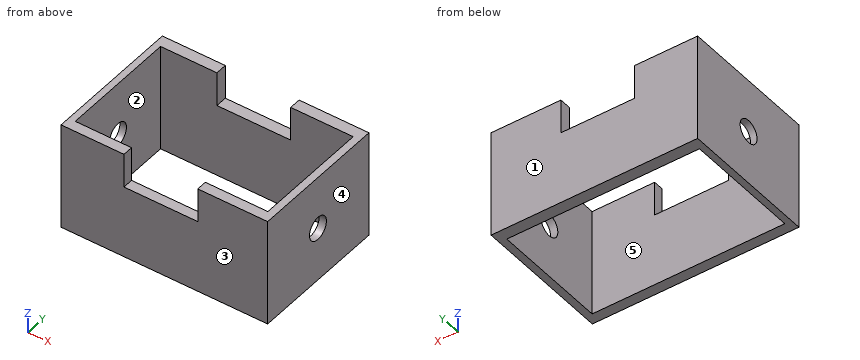
```python
from build123d import *

# Parameters (mm, degrees)
F0_W     = 219.245888
F0_H     = 147.08846
F1_DEPTH = 114.3
F2_W     = 78.317389
F2_H     = 36.511922
F3_DEPTH = 147.089461
F4_W     = 204.472921
F4_H     = 123.958089
F5_DEPTH = 114.301
F6_R     = 12.264791
F7_DEPTH = 219.246888


with BuildPart() as f1:
    # F0 (on Top) → F1 (new body)
    with BuildSketch(Plane.XY):
        with Locations((10.201607, 0.449974)):
            Rectangle(F0_W, F0_H)
    extrude(amount=F1_DEPTH)

    # F2 (on face) → F3 (cut, through all)
    with BuildSketch(Plane.XZ.offset(73.094256)):
        with Locations((6.517709, 96.044039)):
            Rectangle(F2_W, F2_H)
    extrude(amount=-F3_DEPTH, mode=Mode.SUBTRACT)

    # F4 (on face) → F5 (cut, through all)
    with BuildSketch(Plane(origin=(0, 0, 0), x_dir=(1, 0, 0), z_dir=(0, 0, -1))):
        with Locations((9.806979, 0.144809)):
            Rectangle(F4_W, F4_H)
    extrude(amount=-F5_DEPTH, mode=Mode.SUBTRACT)

    # F6 (on face) → F7 (cut, through all)
    with BuildSketch(Plane.YZ.offset(119.824551)):
        with Locations((0, 57.527971)):
            Circle(F6_R)
    extrude(amount=-F7_DEPTH, mode=Mode.SUBTRACT)


solid = f1.part
```
Model file for the job. Use its own axes, mm. Face numbers are marked on the shaded views. A direction names the side the tool comes from. Coordinates: 2 decimals unless noted, no trailing zeros. Order: outer loops, then holes, each group sorted by start corner. A loop starts at its lowest first (then second) coordinate and runs counter-clockwise, first axis right, second up. Notation, with made-up numbers: (75.5, 35.25) - (123.5, 35.25) arc R9 cw to (123.5, 39.25) - close; hole circle Ø9 at (46.25, 65). An arc over 180 degrees is marked (long way). Return JSON: item names as keys, results as strings. Group by question number.
1) Saw through at C-C, the plane z = 75. Write the cut outline in (x, y).
2) Tool access for the marked faces 1 and 2: list every direction of +Z, -Z, +X, -X, +Y, -Y with a clear straight run to the whole face (end or side of a thin tool).
3) Mould opens along X. For the marked faces 3, 4 and 5 say: released by +X, released by -X, zero draft, split by the parting line, or undercut.
4) Saw through at D-D, the plane y = -19. Write the cut outline in (x, z).
5) Probe line 1 (Y direction, x = -80, z = 53); line 2 (X direction, y = -26, z = 67); line 3 (Z direction, x = -96, y = 0). List the from-to ranges inside material, lowest first. Write a range as from..to.
6) Saw through at A-A, the plane y = 0. Write the cut outline in (x, z).
7) Saw through at B-B, the plane x = 74.5. Write the cut outline in (y, z).
8) Flat gauge pin, fed straight in: P1, Ø3.5, axis at x = -8, y = 66, coming from the +Z side. Where does the tip first touch, or does it go through?
Values found:
{
 "1": {"outline": "(-99.42, -73.09) - (119.82, -73.09) - (119.82, 73.99) - (-99.42, 73.99) - close; hole (-92.43, -62.12) - (112.04, -62.12) - (112.04, 61.83) - (-92.43, 61.83) - close"},
 "2": {"face 1": "+Z, -Z, +X, -X, +Y", "face 2": "+Z, -Z"},
 "3": {"face 3": "zero draft", "face 4": "released by +X", "face 5": "undercut"},
 "4": {"outline": "(-99.42, 0) - (-92.43, 0) - (-92.43, 114.3) - (-99.42, 114.3) - close; (112.04, 0) - (119.82, 0) - (119.82, 114.3) - (112.04, 114.3) - close"},
 "5": {"line 1": "y = -73.09..-62.12, 61.83..73.99", "line 2": "x = -99.42..-92.43, 112.04..119.82", "line 3": "z = 0..45.26, 69.79..114.3"},
 "6": {"outline": "(-99.42, 0) - (-92.43, 0) - (-92.43, 45.26) - (-99.42, 45.26) - close; (-99.42, 69.79) - (-92.43, 69.79) - (-92.43, 114.3) - (-99.42, 114.3) - close; (112.04, 0) - (119.82, 0) - (119.82, 45.26) - (112.04, 45.26) - close; (112.04, 69.79) - (119.82, 69.79) - (119.82, 114.3) - (112.04, 114.3) - close"},
 "7": {"outline": "(-73.09, 0) - (-62.12, 0) - (-62.12, 114.3) - (-73.09, 114.3) - close; (61.83, 0) - (73.99, 0) - (73.99, 114.3) - (61.83, 114.3) - close"},
 "8": {"P1": "stops at z = 77.79"}
}
